Design review of the part shown in the three views and the two pictorial views. Dimensions are in mm from the part's minimum x, y and z. Coordinates: 2 decimals unless noted, no trailing zeros. Loops run counter-clockwise (first coordinate to the right, second up) from the corner with the lowest first, then second, coordinate; pieces in that order, holes last.
Q1. Add section A-A on x = 5. Give the boundary of the cut face in (y, z), and give its area (3 significant figures).
Q2. Wall thickness on probe 1 along Y at (x, z) = (26.5, 252); probe 2 along X at (y, z) = (7.25, 183): over which ranges is each line inside the solid? List them lowest first.
Q3. Add section C-C on y = 9. Give the boundary of the cut face in (x, z).
Q4. Add section B-B on z = 48. Give the boundary of the cut face in (x, y), and give its area (3 significant figures).
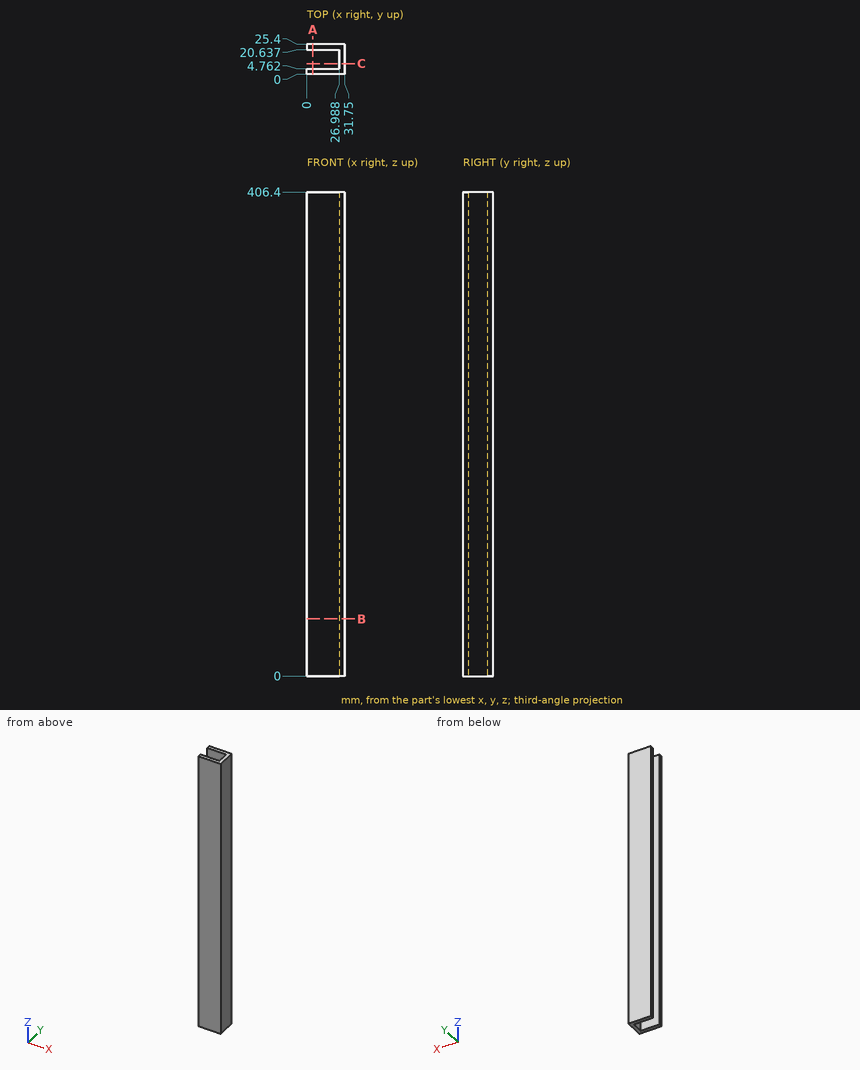
Entries:
1. outline: (0, 0) - (4.76, 0) - (4.76, 406.4) - (0, 406.4) - close; (20.64, 0) - (25.4, 0) - (25.4, 406.4) - (20.64, 406.4) - close
1. area: 3,870 mm2
2. probe 1: y = 0 to 4.76, 20.64 to 25.4
2. probe 2: x = 26.99 to 31.75
3. outline: (26.99, 0) - (31.75, 0) - (31.75, 406.4) - (26.99, 406.4) - close
4. outline: (0, 0) - (31.75, 0) - (31.75, 25.4) - (0, 25.4) - (0, 20.64) - (26.99, 20.64) - (26.99, 4.76) - (0, 4.76) - close
4. area: 378 mm2
